```python
from build123d import *

# Parameters (mm, degrees)
BASE_EXTRUDE_DEPTH = 12.7
CIRPATTERN1_COUNT  = 2
CIRPATTERN1_ANGLE  = 90


with BuildPart() as part:
    # Sketch1 → Base-Extrude (new, symmetric)
    with BuildSketch(Plane.XY):
        with BuildLine():
            Line((-41.275, 39.7764), (-41.275, 34.34565134))
            ThreePointArc((-41.275, 34.34565134), (-39.7764, 31.75), (-41.275, 29.15434866))
            Line((-41.275, 29.15434866), (-41.275, 12.12065134))
            ThreePointArc((-41.275, 12.12065134), (-39.7764, 9.525), (-41.275, 6.92934866))
            Line((-41.275, 6.92934866), (-41.275, 1.4986))
            ThreePointArc((-41.275, 1.4986), (-40.836070222, 0.438929778), (-39.7764, 0))
            Line((-39.7764, 0), (-1.4986, 0))
            ThreePointArc((-1.4986, 0), (-0.438929778, 0.438929778), (0, 1.4986))
            Line((0, 1.4986), (0, 6.92934866))
            ThreePointArc((0, 6.92934866), (-1.4986, 9.525), (0, 12.12065134))
            Line((0, 12.12065134), (0, 29.15434866))
            ThreePointArc((0, 29.15434866), (-1.4986, 31.75), (0, 34.34565134))
            Line((0, 34.34565134), (0, 39.7764))
            ThreePointArc((0, 39.7764), (-0.438929778, 40.836070222), (-1.4986, 41.275))
            Line((-1.4986, 41.275), (-8.0264, 41.275))
            ThreePointArc((-8.0264, 41.275), (-9.086070222, 40.836070222), (-9.525, 39.7764))
            Line((-9.525, 39.7764), (-9.525, 34.925))
            Line((-9.525, 34.925), (-8.0264, 34.925))
            Line((-8.0264, 34.925), (-8.0264, 39.7764))
            Line((-8.0264, 39.7764), (-1.4986, 39.7764))
            Line((-1.4986, 39.7764), (-1.4986, 35.100971471))
            ThreePointArc((-1.4986, 35.100971471), (-2.9972, 31.75), (-1.4986, 28.399028529))
            Line((-1.4986, 28.399028529), (-1.4986, 12.875971471))
            ThreePointArc((-1.4986, 12.875971471), (-2.9972, 9.525), (-1.4986, 6.174028529))
            Line((-1.4986, 6.174028529), (-1.4986, 1.4986))
            Line((-1.4986, 1.4986), (-39.7764, 1.4986))
            Line((-39.7764, 1.4986), (-39.7764, 6.174028529))
            ThreePointArc((-39.7764, 6.174028529), (-38.2778, 9.525), (-39.7764, 12.875971471))
            Line((-39.7764, 12.875971471), (-39.7764, 28.399028529))
            ThreePointArc((-39.7764, 28.399028529), (-38.2778, 31.75), (-39.7764, 35.100971471))
            Line((-39.7764, 35.100971471), (-39.7764, 39.7764))
            Line((-39.7764, 39.7764), (-33.2486, 39.7764))
            Line((-33.2486, 39.7764), (-33.2486, 34.925))
            Line((-33.2486, 34.925), (-31.75, 34.925))
            Line((-31.75, 34.925), (-31.75, 39.7764))
            ThreePointArc((-31.75, 39.7764), (-32.188929778, 40.836070222), (-33.2486, 41.275))
            Line((-33.2486, 41.275), (-39.7764, 41.275))
            ThreePointArc((-39.7764, 41.275), (-40.836070222, 40.836070222), (-41.275, 39.7764))
        make_face()
    base_extrude = extrude(amount=BASE_EXTRUDE_DEPTH, both=True)

    # CirPattern1: Base-Extrude ×2 about axis
    cirpattern1_axis = Axis((0, 0, 0), (0, 0, 1))
    for i in range(1, CIRPATTERN1_COUNT):
        add(base_extrude.rotate(cirpattern1_axis, i * CIRPATTERN1_ANGLE / (CIRPATTERN1_COUNT - 1)))


solid = part.part
```
Part model, mm, in its own coordinate system. A direction names the side the tool comes from. Round coordinates to 2 decimals unless told otherwise and drop trailing zeros. Order: outer loops, then holes, each group sorted by start corner. A loop starts at its lowest first (then second) coordinate and runs counter-clockwise, first axis right, second up. Notation, with made-up numbers: M -19.5,-16 L 4.5,-16 A34 ccw 4.5,22 Z; hole C -8,61.25 d4. An arc over 180 degrees is marked long. Put each result on its own line as item: value. Start each with the question number.
1. Slice it at B-B on z = -9. State how many separate pieces and enclosed holes the cut face has, then the cut area to 3 significant figures.
2. Drill centre lines: probe 1 along Y at (x, z) = (-5.5, -9.5) (3 decimals); probe 2 along Y at (x, z) = (-35.5, 11.5) (3 decimals); probe 3 along Y at (x, z) = (-24, -9) (3 decimals). Where is each one in solid material? Low to high. Write a range as [from, to].
3. Slice it at A-A on y = 23.5. List the corners of the cut face in (x, z) (3 decimals).
4. Two-plate mould, pull along Y, no slides. Class faces 3 (the face through (-19, 0, 12.7)), 4 (the face through (-4, -39.776, 0)), 5 (the face through (-4, -41.275, 0)): +Y half, -Y half, draft (parallel to the pull), parting line (faces both ways), or undercut.
5. Tool access for faces 1 (the face through (-37, -1.499, 0)), 2 (the face through (-1.5, 31.7, 0.2)): list every direction of +Z, -Z, +X, -X, +Y, -Y with a clear straight run to the whole face (end or side of a thin tool).
6. Slice it at C-C on y = -26.5. List the corners of the cut face in (x, z), then the cut area to 3 significant figures.
7. Drop flat-ended pins along their axis: pin 1 (2 mm diameter, centred on y = 30.5, z = 7.5, fed in from +X); pin 2 (6 mm diameter, centred on x = -18.5, z = -6, fed in from +Y). Give the stop position or say it passes through.
Findings:
1. separate pieces: 1
1. enclosed holes: 2
1. area: 445 mm2
2. probe 1: [-41.275, -39.776], [-1.499, 1.499], [39.776, 41.275]
2. probe 2: [-41.275, -39.776], [-33.249, -31.75], [-9.525, -8.026], [-1.499, 1.499], [39.776, 41.275]
2. probe 3: [-41.275, -39.776], [-1.499, 1.499]
3. outline: M -41.275,-12.7 L -39.776,-12.7 L -39.776,12.7 L -41.275,12.7 Z; M -1.499,-12.7 L 0,-12.7 L 0,12.7 L -1.499,12.7 Z
4. face 3: draft
4. face 4: undercut
4. face 5: -Y half
5. face 1: +Z, -Z
5. face 2: +Z, -Z, +X
6. outline: M -1.5,-12.7 L 0,-12.7 L 0,12.7 L -1.5,12.7 Z
6. area: 38.1 mm2
7. pin 1: x = -0.48
7. pin 2: y = 1.5
